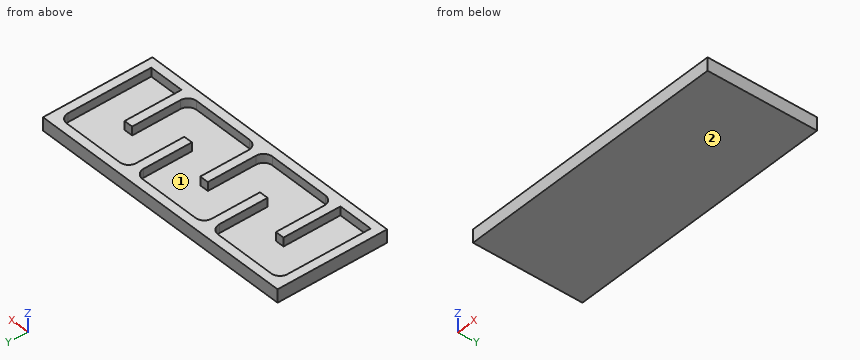
from build123d import *

# Parameters (mm, degrees)
F0_W     = 62
F0_H     = 25
F1_DEPTH = 1
F2_W     = 62
F2_H     = 25
F3_DEPTH = 2


# Not quite as in the source:
# - a feature names something its author has since deleted; it is built from what else it names


with BuildPart() as f1:
    # F0 (on Top) → F1 (new body)
    with BuildSketch(Plane.XY):
        Rectangle(F0_W, F0_H)
    extrude(amount=F1_DEPTH)

    # F2 (on face) → F3 (join)
    with BuildSketch(Plane.XY.offset(1)):
        Rectangle(F2_W, F2_H)
        with BuildLine():
            ThreePointArc((-29, 8.5), (-28.4142135624, 9.9142135624), (-27, 10.5))
            Line((-27, 10.5), (-13, 10.5))
            ThreePointArc((-13, 10.5), (-11.5857864376, 9.9142135624), (-11, 8.5))
            Line((-11, 8.5), (-11, -2.5))
            Line((-11, -2.5), (-9, -2.5))
            Line((-9, -2.5), (-9, 8.5))
            ThreePointArc((-9, 8.5), (-8.4142135624, 9.9142135624), (-7, 10.5))
            Line((-7, 10.5), (7, 10.5))
            ThreePointArc((7, 10.5), (8.4142135624, 9.9142135624), (9, 8.5))
            Line((9, 8.5), (9, -2.5))
            Line((9, -2.5), (11, -2.5))
            Line((11, -2.5), (11, 8.5))
            ThreePointArc((11, 8.5), (11.5857864376, 9.9142135624), (13, 10.5))
            Line((13, 10.5), (27, 10.5))
            ThreePointArc((27, 10.5), (28.4142135624, 9.9142135624), (29, 8.5))
            Line((29, 8.5), (29, -10.5))
            Line((29, -10.5), (21, -10.5))
            Line((21, -10.5), (21, 2.5))
            Line((21, 2.5), (19, 2.5))
            Line((19, 2.5), (19, -8.5))
            ThreePointArc((19, -8.5), (18.4142135624, -9.9142135624), (17, -10.5))
            Line((17, -10.5), (3, -10.5))
            ThreePointArc((3, -10.5), (1.5857864376, -9.9142135624), (1, -8.5))
            Line((1, -8.5), (1, 2.5))
            Line((1, 2.5), (-1, 2.5))
            Line((-1, 2.5), (-1, -8.5))
            ThreePointArc((-1, -8.5), (-1.5857864376, -9.9142135624), (-3, -10.5))
            Line((-3, -10.5), (-17, -10.5))
            ThreePointArc((-17, -10.5), (-18.4142135624, -9.9142135624), (-19, -8.5))
            Line((-19, -8.5), (-19, 2.5))
            Line((-19, 2.5), (-21, 2.5))
            Line((-21, 2.5), (-21, -10.5))
            Line((-21, -10.5), (-29, -10.5))
            Line((-29, -10.5), (-29, 8.5))
        make_face(mode=Mode.SUBTRACT)
    extrude(amount=F3_DEPTH)


solid = f1.part
Work out the finished part from the listing and answer in its coordinate system (mm). Face numbers are marked on the shaded views. Round coordinates to 2 decimals unless told otherwise and drop trailing zeros. Write each loop counter-clockwise with the first axis right and the second up, starting at its lowest first coordinate (ties: lowest second). Pieces come first, ordered by that corner, then holes. Notation, with made-up numbers: (-12.75, -37.75) - (36.25, -37.75) arc R18 ccw to (36.25, -23.75) - close; hole circle Ø10 at (67.25, 59). An arc over 180 degrees is marked (long way). Answer in a Markdown table with one row per item. Add a question column.
1. Find the intervals of material crossed by line 1 along X through (y, z) = (-7.75, 2.25); line 2 along Y through (x, z) = (10, 2.8); line 3 along X through (y, z) = (6.75, 2.8), in increasing order. Write a range as from..to.
2. A cutting plane is placed at C-C, the plane y = 4.5. Determine the outline of the cut face in (x, z).
3. The mould has two halves that part along Y. Classify the marked faces 1 and 2: +Y half, -Y half, draft (parallel to the pull), parting line (faces both ways), or undercut.
4. A cutting plane is placed at D-D, the plane y = -0.25. Determine the outline of the cut face in (x, z), and give its area (3 significant figures).
5. A cutting plane is placed at B-B, the plane x = 24. Determine the outline of the cut face in (y, z), and give its area (3 significant figures).
6. A cutting plane is placed at A-A, the plane y = -7. Determine the outline of the cut face in (x, z).
7. Given pin 1 (4 mm diameter, centred on x = -24.5, y = -3, fed in from +Z), flat-ended and moving along its own axis, determine where the tip first touches the part or whether it passes through.
Worked out:
| question | item | result |
|---|---|---|
| 1 | line 1 | -31..-29, -21..-19, -1..1, 19..21, 29..31 |
| 1 | line 2 | -12.5..-10.5, -2.5..12.5 |
| 1 | line 3 | -31..-29, -11..-9, 9..11, 29..31 |
| 2 | outline | (-31, 0) - (31, 0) - (31, 3) - (29, 3) - (29, 1) - (11, 1) - (11, 3) - (9, 3) - (9, 1) - (-9, 1) - (-9, 3) - (-11, 3) - (-11, 1) - (-29, 1) - (-29, 3) - (-31, 3) - close |
| 3 | face 1 | undercut |
| 3 | face 2 | draft |
| 4 | outline | (-31, 0) - (31, 0) - (31, 3) - (29, 3) - (29, 1) - (21, 1) - (21, 3) - (19, 3) - (19, 1) - (11, 1) - (11, 3) - (9, 3) - (9, 1) - (1, 1) - (1, 3) - (-1, 3) - (-1, 1) - (-9, 1) - (-9, 3) - (-11, 3) - (-11, 1) - (-19, 1) - (-19, 3) - (-21, 3) - (-21, 1) - (-29, 1) - (-29, 3) - (-31, 3) - close |
| 4 | area | 90.0 mm^2 |
| 5 | outline | (-12.5, 0) - (12.5, 0) - (12.5, 3) - (10.5, 3) - (10.5, 1) - (-10.5, 1) - (-10.5, 3) - (-12.5, 3) - close |
| 5 | area | 33.0 mm^2 |
| 6 | outline | (-31, 0) - (31, 0) - (31, 3) - (29, 3) - (29, 1) - (21, 1) - (21, 3) - (19, 3) - (19, 1) - (1, 1) - (1, 3) - (-1, 3) - (-1, 1) - (-19, 1) - (-19, 3) - (-21, 3) - (-21, 1) - (-29, 1) - (-29, 3) - (-31, 3) - close |
| 7 | pin 1 | z = 1 |
